The figure shows three views and two pictorial views of one solid part (mm, origin at its lowest corner). Answer the questions. A direction names the side the tool comes from. Coordinates: 2 decimals unless noted, no trailing zeros. Loops run counter-clockwise (first coordinate to the right, second up) from the corner with the lowest first, then second, coordinate; pieces in that order, holes last.
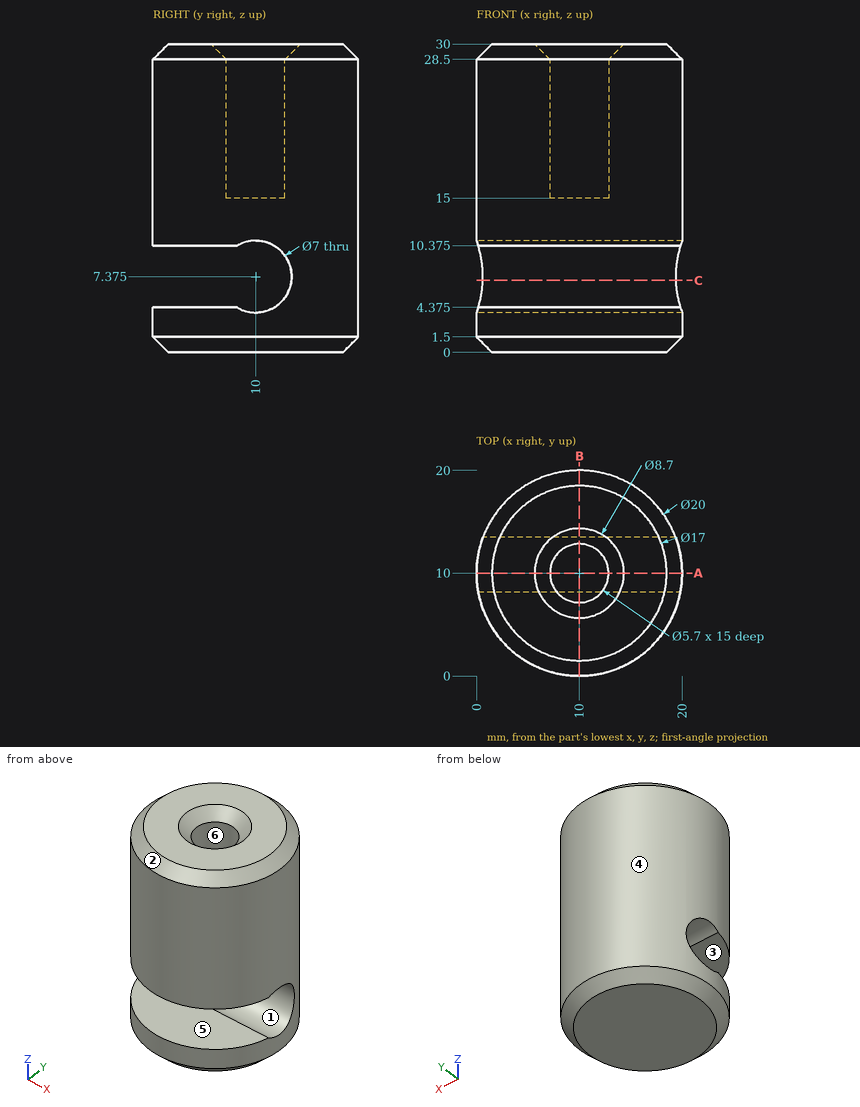
Q1. Which of the six approach directions +Z, -Z, +X, -X, +Y, -Y give full straight-line access (tool end or side, diameter ignored) to the marked faces 4, 5 and 6?
Findings below:
face 4: +Z, -Z
face 5: +X, -X, -Y
face 6: +Z
Q2. A cutting plane is placed at A-A (y = 10). Give the vertices of the cut face in (x, z) (3 decimals).
Findings below:
outline: (0, 1.5) - (1.5, 0) - (18.5, 0) - (20, 1.5) - (20, 3.875) - (0, 3.875) - close; (0, 10.875) - (20, 10.875) - (20, 28.5) - (18.5, 30) - (14.35, 30) - (12.85, 28.5) - (12.85, 15) - (7.15, 15) - (7.15, 28.5) - (5.65, 30) - (1.5, 30) - (0, 28.5) - close
Q3. Flat-ended cylindrical pins translate along their axes: pin 1 Ø4 at (y, z) = (17.5, 22.5) entering from -X; pin 2 Ø12 at (x, y) = (10, 3.5) entering from -Z; pin 3 Ø3 at (x, y) = (11, 10.5) entering from +Z; pin 4 Ø6 at (x, z) = (15, 11.5) entering from +Y. Find the tip coordinate at first contact, or state that the pin passes through.
Findings below:
pin 1: stops at x = 1.65
pin 2: stops at z = 0
pin 3: stops at z = 15
pin 4: stops at y = 19.8
Q4. Straight lines are drawn through the part: probe 1 along Z at (x, y) = (10.25, 10) (3 decimals); probe 2 along Z at (x, y) = (12.25, 4) (3 decimals); probe 3 along Y at (x, z) = (10, 21.75). For each, find the intervals that lie inside material, in ascending order.
Findings below:
probe 1: z = 0 to 3.875, 10.875 to 15
probe 2: z = 0 to 4.375, 10.375 to 30
probe 3: y = 0 to 7.15, 12.85 to 20
Q5. A cutting plane is placed at C-C (z = 7). Give the vertices of the cut face in (x, y) (3 decimals).
Findings below:
outline: (0.625, 13.48) - (19.375, 13.48) arc R10 ccw to start
Q6. Determine the mould class of the marked faces 1, 2 and 3 for opening direction Y: +Y half, -Y half, draft (parallel to the pull), parting line (faces both ways), or undercut.
Findings below:
face 1: undercut
face 2: parting line
face 3: draft
Q7. A cutting plane is placed at B-B (x = 10). Give the vertices of the cut face in (y, z) (3 decimals), then the cut area to 3 significant figures.
Findings below:
outline: (0, 1.5) - (1.5, 0) - (18.5, 0) - (20, 1.5) - (20, 28.5) - (18.5, 30) - (14.35, 30) - (12.85, 28.5) - (12.85, 15) - (7.15, 15) - (7.15, 28.5) - (5.65, 30) - (1.5, 30) - (0, 28.5) - (0, 10.375) - (8.197, 10.375) arc R3.5 cw (long way) to (8.197, 4.375) - (0, 4.375) - close
area: 427 mm2
